For this review, take the finished solid that the model builds, in its own axes (mm). Coordinates: 2 decimals unless noted, no trailing zeros. Order: outer loops, then holes, each group sorted by start corner. A loop starts at its lowest first (then second) coordinate and runs counter-clockwise, first axis right, second up. Notation, with made-up numbers: (11, 8.25) -> (48, 8.25) arc R14 cw to (48, 33.25) -> close; hole circle Ø2 at (-40, 68.25). An arc over 180 degrees is marked (long way). Return JSON: item names as keys, results as strings. Group by question number.
Item 1: Take a section at A-A (z = -1.75). Write out the cut boundary in (x, y), then the cut area to 3 significant figures.
Item 2: Take a section at B-B (z = 2). Write out the cut boundary in (x, y) (3 decimals).
Item 3: For line 1 along X through (y, z) = (0.1, 2); line 2 along Y through (x, z) = (-0.4, 6.5), list the stretches that pass through material, from the lowest coordinate up.
Item 4: Draft analysis for pull direction Z (two halves, no side actions). For faces 1 (the cylindrical face through (-1.474, 0.065, 3.944)), 2 (the cylindrical face through (0.194, 1.477, -1.38)), 3 (the flat face through (0, 0, -2.9)), state which applies: +Z half, -Z half, draft (parallel to the pull), parting line (faces both ways), or undercut.
Item 5: Insertion check: pin 1 (1.5 mm diameter, centred on y = -0.5, z = 8, fed in from +X). The pin has a flat end and moves straight along its axis. Give the tip position at first contact, or say it passes through.
```python
from build123d import *

# Parameters (mm, degrees)
SKETCH_1_R      = 1.475
EXTRUDE_1_DEPTH = 8
SKETCH_2_R      = 1.49
EXTRUDE_2_DEPTH = 2.9
EXTRUDE_START   = 2.9
SKETCH_3_R      = 1.49
EXTRUDE_3_DEPTH = 2.9
CHAMFER_1_SIZE  = 0.1


with BuildPart() as part:
    # 스케치1 → 보스-돌출1 (new body)
    with BuildSketch(Plane.XY):
        Circle(SKETCH_1_R)
    extrude(amount=EXTRUDE_1_DEPTH)

    # 스케치2 → 보스-돌출2 (add)
    with BuildSketch(Plane(origin=(0, 0, 0), x_dir=(-1, 0, 0), z_dir=(0, 0, -1))):
        Circle(SKETCH_2_R)
    extrude(amount=EXTRUDE_2_DEPTH)

    # 스케치3 → 보스-돌출3 (add)
    with BuildSketch(Plane.XY.offset(8).offset(EXTRUDE_START)):
        with Locations(Location((0, 0, 0), (0, 0, 180))):
            Circle(SKETCH_3_R)
    extrude(amount=-EXTRUDE_3_DEPTH)

    # 모따기1
    chamfer_1_edges = [part.edges().sort_by_distance(p)[0] for p in [
        (1.49, 0, -2.9),
        (1.49, 0, 10.9),
    ]]
    chamfer(chamfer_1_edges, length=CHAMFER_1_SIZE)


solid = part.part
```
Findings below:
{
 "1": {"outline": "circle Ø2.98 at (0, 0)", "area": "6.97 mm2"},
 "2": {"outline": "circle Ø2.95 at (0, 0)"},
 "3": {"line 1": "x = -1.47 to 1.47", "line 2": "y = -1.42 to 1.42"},
 "4": {"face 1": "undercut", "face 2": "draft", "face 3": "-Z half"},
 "5": {"pin 1": "stops at x = 1.49"}
}
